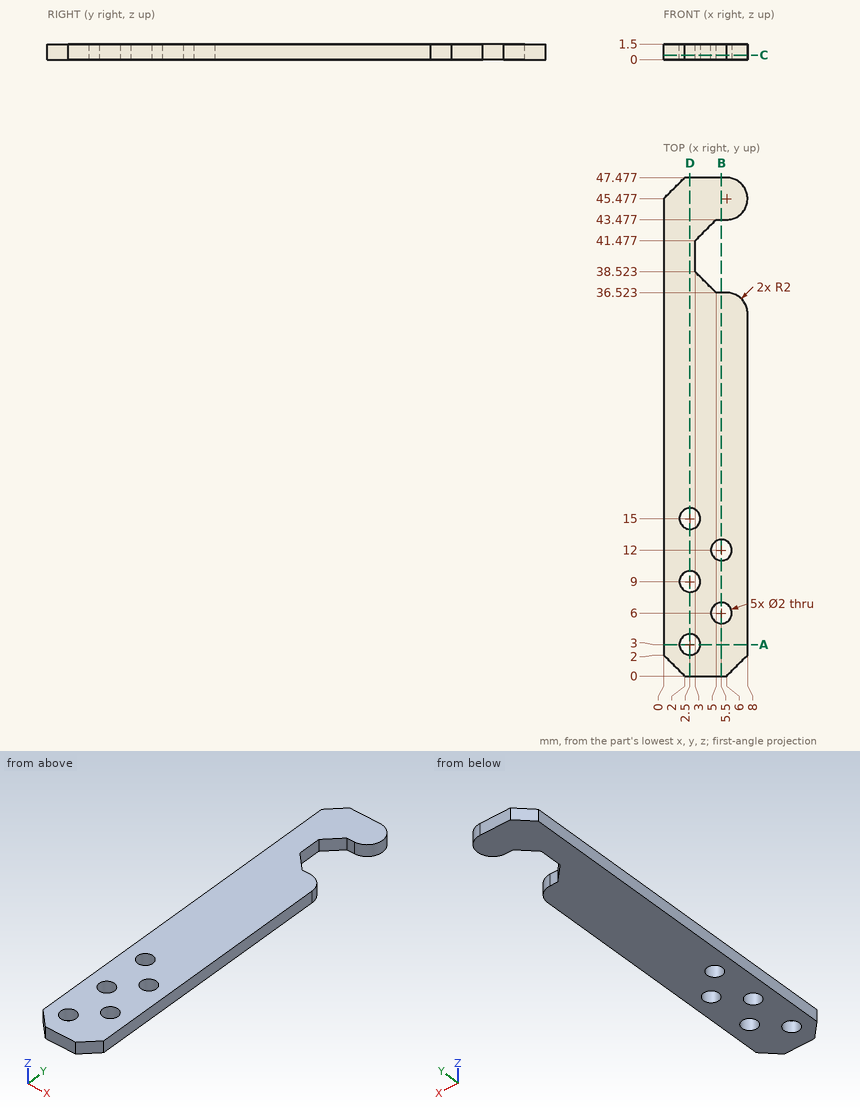
Print and shaded views of the part. All mm, measured from the part's lowest x, y and z. Give positions to 0.01 mm unless a question says otherwise; leave off trailing zeros. Order: outer loops, then holes, each group sorted by start corner. A loop starts at its lowest first (then second) coordinate and runs counter-clockwise, first axis right, second up. Notation, with made-up numbers: M 14,51 L 47,51 A21 ccw 47,61 Z; hole C 14,-17 d9. An arc over 180 degrees is marked long. Use one line per item in the form item = value.
Q1. Slice it at B-B, the plane x = 5.5. Write the cut outline in (y, z).
Conclusion:
outline = M 0,0 L 5,0 L 5,1.5 L 0,1.5 Z; M 7,0 L 11,0 L 11,1.5 L 7,1.5 Z; M 13,0 L 36.52,0 L 36.52,1.5 L 13,1.5 Z; M 43.48,0 L 47.48,0 L 47.48,1.5 L 43.48,1.5 Z
Q2. Slice it at D-D, the plane x = 2.5. Write the cut outline in (y, z).
Conclusion:
outline = M 0,0 L 2,0 L 2,1.5 L 0,1.5 Z; M 4,0 L 8,0 L 8,1.5 L 4,1.5 Z; M 10,0 L 14,0 L 14,1.5 L 10,1.5 Z; M 16,0 L 47.48,0 L 47.48,1.5 L 16,1.5 Z
Q3. Slice it at C-C, the plane z = 0.45. Write the cut outline in (x, y).
Conclusion:
outline = M 0,2 L 2,0 L 6,0 L 8,2 L 8,34.52 A2 ccw 6,36.52 L 5,36.52 L 3,38.52 L 3,41.48 L 5,43.48 L 6,43.48 A2 ccw 6,47.48 L 2,47.48 L 0,45.48 Z; hole C 2.5,3 d2; hole C 2.5,9 d2; hole C 2.5,15 d2; hole C 5.5,6 d2; hole C 5.5,12 d2
Q4. Slice it at A-A, the plane y = 3. Write the cut outline in (x, z).
Conclusion:
outline = M 0,0 L 1.5,0 L 1.5,1.5 L 0,1.5 Z; M 3.5,0 L 8,0 L 8,1.5 L 3.5,1.5 Z
Q5. Pin check, flat tips, straight feed: P1, Ø2.5, axis at x = 5.5, y = 6, coming from the -Z side; P2, Ø1.6, axis at x = 2.5, y = 15, coming from the -Z side. Stop position of each tip, or through.
Conclusion:
P1 = 0
P2 = through
Q6. Wall check: probe 1 along Y at (x, z) = (2.5, 1.1); probe 2 along Y at (x, z) = (5.5, 0.4); probe 3 along X at (y, z) = (6, 0.95). Give the ranges that are in metal, low to high.
Conclusion:
probe_1 = 0 to 2, 4 to 8, 10 to 14, 16 to 47.48
probe_2 = 0 to 5, 7 to 11, 13 to 36.52, 43.48 to 47.48
probe_3 = 0 to 4.5, 6.5 to 8
